from build123d import *

# Parameters (mm, degrees)
SKIZZE1_W                                 = 25
SKIZZE1_H                                 = 24
PCB_DEPTH                                 = 0.9
SKIZZE2_R                                 = 1.05
MOUNTING_HOLES_DEPTH                      = 1.9
SKIZZE3_W                                 = 20.8
SKIZZE3_H                                 = 5.5
CONNECTOR_CLOSED_DEPTH                    = 2.4
SKIZZE4_W                                 = 17.7
SKIZZE4_H                                 = 11.6
COMPONENTS_WORST_CASE_BOUNDARY_BOX_DEPTH  = 1.3
SKIZZE7_W                                 = 3
SKIZZE7_H                                 = 2
COMPONENTS_WORST_CASE_BOUNDARY_BOX2_DEPTH = 0.6
SKIZZE8_W                                 = 1.3
SKIZZE8_H                                 = 0.9
STATUS_LED_DEPTH                          = 0.01


with BuildPart() as part:
    # Skizze1 → PCB (new body)
    with BuildSketch(Plane(origin=(0, 0, 0), x_dir=(1, 0, 0), z_dir=(0, 1, 0))):
        with Locations((0, 2.5)):
            Rectangle(SKIZZE1_W, SKIZZE1_H)
    extrude(amount=-PCB_DEPTH)

    # Skizze2 → Mounting_Holes (cut, through all)
    with BuildSketch(Plane(origin=(0, 0, 0), x_dir=(1, 0, 0), z_dir=(0, 1, 0))):
        with Locations((10.5, 12.5)):
            Circle(SKIZZE2_R)
        with Locations((10.5, 0)):
            Circle(SKIZZE2_R)
        with Locations((-10.5, 0)):
            Circle(SKIZZE2_R)
        with Locations((-10.5, 12.5)):
            Circle(SKIZZE2_R)
    extrude(amount=-MOUNTING_HOLES_DEPTH, mode=Mode.SUBTRACT)

    # Skizze3 → Connector_closed (add)
    with BuildSketch(Plane.XZ.offset(0.9)):
        with Locations((0, 6.75)):
            Rectangle(SKIZZE3_W, SKIZZE3_H)
    extrude(amount=CONNECTOR_CLOSED_DEPTH)

    # Skizze4 → Components_worst-case_Boundary-Box (add)
    with BuildSketch(Plane.XZ.offset(0.9)):
        with Locations((-0.15, -6.7)):
            Rectangle(SKIZZE4_W, SKIZZE4_H)
    extrude(amount=COMPONENTS_WORST_CASE_BOUNDARY_BOX_DEPTH)

    # Skizze7 → Components_worst-case_Boundary-Box2 (add)
    with BuildSketch(Plane(origin=(0, 0, 0), x_dir=(1, 0, 0), z_dir=(0, 1, 0))):
        with Locations((7, 9.9)):
            Rectangle(SKIZZE7_W, SKIZZE7_H)
    extrude(amount=COMPONENTS_WORST_CASE_BOUNDARY_BOX2_DEPTH)

    # Skizze8 → Status_LED (cut)
    with BuildSketch(Plane(origin=(0, 0.6, 0), x_dir=(1, 0, 0), z_dir=(0, 1, 0))):
        with Locations((7.45, 9.45)):
            Rectangle(SKIZZE8_W, SKIZZE8_H)
    extrude(amount=-STATUS_LED_DEPTH, mode=Mode.SUBTRACT)


solid = part.part
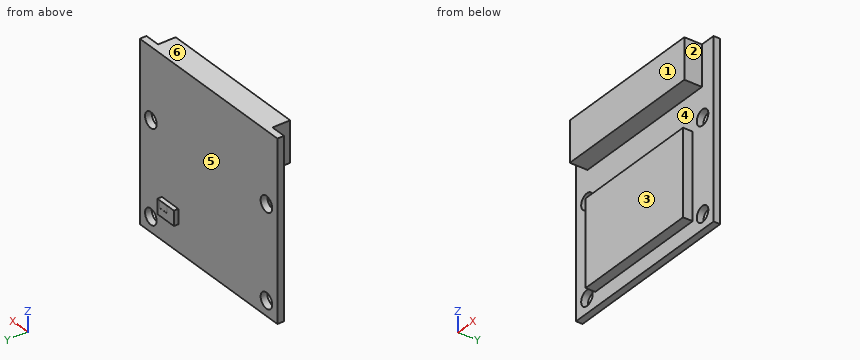
For this review, take the finished solid that the model builds, in its own axes (mm). Face numbers are marked on the shaded views. A direction names the side the tool comes from. Round coordinates to 2 decimals unless told otherwise and drop trailing zeros. Loops run counter-clockwise (first coordinate to the right, second up) from the corner with the lowest first, then second, coordinate; pieces in that order, holes last. Notation, with made-up numbers: (42.25, 88) - (54.25, 88) arc R26 ccw to (54.25, 109) - close; hole circle Ø3 at (29.5, -6.75). An arc over 180 degrees is marked (long way). Answer as CSV lines item,"result".
(1) Consider section B-B on z = 0. Give the boundary of the cut face in (x, y), then the cut area to 3 significant figures.
Checked values:
outline,"(-12.5, -0.9) - (-11.55, -0.9) - (-11.55, 0) - (-12.5, 0) - close; (-9.45, -0.9) - (9.45, -0.9) - (9.45, 0) - (-9.45, 0) - close; (11.55, -0.9) - (12.5, -0.9) - (12.5, 0) - (11.55, 0) - close"
area,"18.7 mm2"
(2) Consider section A-A on y = -1.75. Give the boundary of the cut face in (x, z), then the cut area to 3 significant figures.
Checked values:
outline,"(-10.4, 4) - (10.4, 4) - (10.4, 9.5) - (-10.4, 9.5) - close; (-9, -12.5) - (8.7, -12.5) - (8.7, -0.9) - (-9, -0.9) - close"
area,"320 mm2"
(3) Wall thickness on line 1 (X direction, y = -0.35, z = -12.5); line 2 (Z direction, x = 10.5, y = -0.2); line 3 (Z direction, x = 10.25, y = -3): over which ranges is each line inside the solid? List them lowest first.
Checked values:
line 1,"x = -12.5 to -11.55, -9.45 to 9.45, 11.55 to 12.5"
line 2,"z = -14.5 to -13.55, -11.45 to -1.05, 1.05 to 9.5"
line 3,"z = 4 to 9.5"
(4) Tool access review of the marked faces 1, 2 and 3: name each direction out of +Z, -Z, +X, -X, +Y, -Y from which nothing blocks a thin tool from reaching the whole face with its end or side.
Checked values:
face 1,"+Z, -Z, +X, -X, -Y"
face 2,"+Z, -Z, +X, -Y"
face 3,"-Z, +X, -X, -Y"
(5) Mouldability with a two-part tool opening along Z and no side actions: class the marked faces 4, 5 and 6 as +Z half, -Z half, draft (parallel to the pull), parting line (faces both ways), or undercut.
Checked values:
face 4,"undercut"
face 5,"draft"
face 6,"+Z half"
(6) Consider section C-C on x = -5.25. Give the boundary of the cut face in (y, z), then the cut area to 3 significant figures.
Checked values:
outline,"(-3.3, 4) - (-0.9, 4) - (-0.9, -0.9) - (-2.2, -0.9) - (-2.2, -12.5) - (-0.9, -12.5) - (-0.9, -14.5) - (0, -14.5) - (0, 9.5) - (-3.3, 9.5) - close"
area,"49.9 mm2"
(7) Insertion check: P1, Ø2, axis at x = -8.5, z = 2.5, coming from the -Y side; P2, Ø7, axis at x = -5.5, z = -7.5, coming from the +Y side; P3, Ø1, axis at y = -1.5, z = -7, coming from the -X side. Each pin has a flat end and moves straight along its axis. Give the tip position at first contact, or say it passes through.
Checked values:
P1,"stops at y = -0.9"
P2,"stops at y = 0"
P3,"stops at x = -9"
(8) Consider section D-D on z = 7.25. Give the boundary of the cut face in (x, y).
Checked values:
outline,"(-12.5, -0.9) - (-10.4, -0.9) - (-10.4, -3.3) - (10.4, -3.3) - (10.4, -0.9) - (12.5, -0.9) - (12.5, 0) - (-12.5, 0) - close"
